```python
from build123d import *

# Parameters (mm, degrees)
SKETCH2_R           = 1.651
BOSS_EXTRUDE2_DEPTH = 6.35
FILLET2_R           = 20.32
FILLET3_R           = 2.54


with BuildPart() as part:
    # Sketch2 → Boss-Extrude2 (new body)
    with BuildSketch(Plane(origin=(0, 0, 0), x_dir=(0, 0, -1), z_dir=(1, 0, 0))):
        with BuildLine():
            Line((-22.16, -6.6675), (-22.16, -44.45))
            ThreePointArc((-22.16, -44.45), (0, -66.61), (22.16, -44.45))
            Line((22.16, -44.45), (22.16, 44.45))
            ThreePointArc((22.16, 44.45), (0, 66.61), (-22.16, 44.45))
            Line((-22.16, 44.45), (-22.16, 6.6675))
            Line((-22.16, 6.6675), (-126.3, 6.6675))
            Line((-126.3, 6.6675), (-126.3, -6.6675))
            Line((-126.3, -6.6675), (-22.16, -6.6675))
        make_face()
        with BuildLine():
            ThreePointArc((12, -44.45), (0, -56.45), (-12, -44.45))
            Line((-12, -44.45), (-12, 44.45))
            ThreePointArc((-12, 44.45), (0, 56.45), (12, 44.45))
            Line((12, 44.45), (12, -44.45))
        make_face(mode=Mode.SUBTRACT)
        with Locations((-111.06, 0)):
            Circle(SKETCH2_R, mode=Mode.SUBTRACT)
        with Locations((-103.44, 0)):
            Circle(SKETCH2_R, mode=Mode.SUBTRACT)
        with Locations((-118.68, 0)):
            Circle(SKETCH2_R, mode=Mode.SUBTRACT)
    extrude(amount=BOSS_EXTRUDE2_DEPTH)

    # Fillet2
    fillet2_edges = [part.edges().sort_by_distance(p)[0] for p in [
        (3.175, 6.6675, 22.16),
        (3.175, -6.6675, 22.16),
    ]]
    fillet(fillet2_edges, radius=FILLET2_R)

    # Fillet3
    fillet3_edges = [part.edges().sort_by_distance(p)[0] for p in [
        (3.175, 6.6675, 126.3),
        (3.175, -6.6675, 126.3),
    ]]
    fillet(fillet3_edges, radius=FILLET3_R)


solid = part.part
```
Check sheet for the modelled part. Datum: model origin and axes. Units: mm. A direction names the side the tool comes from. Give positions to 0.01 mm unless a question says otherwise; leave off trailing zeros. Order: outer loops, then holes, each group sorted by start corner. A loop starts at its lowest first (then second) coordinate and runs counter-clockwise, first axis right, second up. Notation, with made-up numbers: (73, 61) -> (114, 61) arc R18 cw to (114, 72) -> close; hole circle Ø2 at (-37, 37.25). An arc over 180 degrees is marked (long way). Use CSV: the item, a comma, the result in double quotes. Start each with the question number.
1) Sectioned sample at A-A, the plane z = 111.06. Record the boundary of the cut face in (x, y).
2) Set-up check for faces 1 (the face through (3, 0, 126.3)), 2 (the face through (0, 0, 25)), 3 (the face through (3, -36, 22.16)), 4 (the face through (3.131, -56.447, -0.264)), 5 (the face through (3, 36, 22.16)): record each of +Z, -Z, +X, -X, +Y, -Y from which the full face is reachable in a straight line by a thin tool's end or side.
3) Sectioned sample at D-D, the plane y = 0. Record the boundary of the cut face in (x, z), plus the area to 3 significant figures.
4) Sectioned sample at B-B, the plane y = -34.5. Record the boundary of the cut face in (x, z), plus the area to 3 significant figures.
5) Mould release check, pull along Z, two halves, no side actions. Record for faces 6 (the face through (3, 1, -12)), 7 (the face through (3, 6.668, 83)), 8 (the face through (3.22, -12.78, 27.95)): released by +Z, released by -Z, zero draft, split by the parting line, or undercut.
6) Material ranges on line 1 (Z direction, x = 4.5, y = -40.5); line 2 (Y direction, x = 3, z = 51); line 3 (Y direction, x = 4.5, z = 111.06), recorded low to high. Write a range as from..to.
7) Sectioned sample at C-C, the plane x = 3.75. Record the boundary of the cut face in (y, z).
8) Go/stop test with flat-tipped pins: P1, Ø2, axis at y = 0, z = 111.06, coming from the +X side; P2, Ø1.9, axis at x = 2, z = 80, coming from the -Y side; P3, Ø3, axis at x = 2.5, y = 33.5, coming from the +Z side; P4, Ø1.9, axis at x = 2, y = 18, coming from the +Z side. Record where each tip stops, or that it passes through.
Recorded:
1,outline,"(0, -6.67) -> (6.35, -6.67) -> (6.35, -1.65) -> (0, -1.65) -> close; (0, 1.65) -> (6.35, 1.65) -> (6.35, 6.67) -> (0, 6.67) -> close"
2,face 1,"+Z, +X, -X, +Y, -Y"
2,face 2,"+Z, -Z, -X, +Y, -Y"
2,face 3,"+Z, +X, -X, -Y"
2,face 4,"+X, -X"
2,face 5,"+Z, +X, -X, +Y"
3,outline,"(0, -22.16) -> (6.35, -22.16) -> (6.35, -12) -> (0, -12) -> close; (0, 12) -> (6.35, 12) -> (6.35, 101.79) -> (0, 101.79) -> close; (0, 105.09) -> (6.35, 105.09) -> (6.35, 109.41) -> (0, 109.41) -> close; (0, 112.71) -> (6.35, 112.71) -> (6.35, 117.03) -> (0, 117.03) -> close; (0, 120.33) -> (6.35, 120.33) -> (6.35, 126.3) -> (0, 126.3) -> close"
3,area,"727 mm2"
4,outline,"(0, -22.16) -> (6.35, -22.16) -> (6.35, -12) -> (0, -12) -> close; (0, 12) -> (6.35, 12) -> (6.35, 22.16) -> (0, 22.16) -> close"
4,area,"129 mm2"
5,face 6,"undercut"
5,face 7,"zero draft"
5,face 8,"released by +Z"
6,line 1,"-22.16..-12, 12..22.16"
6,line 2,"-6.67..6.67"
6,line 3,"-6.67..-1.65, 1.65..6.67"
7,outline,"(-44.45, -22.16) -> (44.45, -22.16) arc R22.16 ccw to (44.45, 22.16) -> (26.99, 22.16) arc R20.32 cw to (6.67, 42.48) -> (6.67, 123.76) arc R2.54 ccw to (4.13, 126.3) -> (-4.13, 126.3) arc R2.54 ccw to (-6.67, 123.76) -> (-6.67, 42.48) arc R20.32 cw to (-26.99, 22.16) -> (-44.45, 22.16) arc R22.16 ccw to start; hole (-44.45, -12) -> (44.45, -12) arc R12 ccw to (44.45, 12) -> (-44.45, 12) arc R12 ccw to start; hole circle Ø3.3 at (0, 103.44); hole circle Ø3.3 at (0, 111.06); hole circle Ø3.3 at (0, 118.68)"
8,P1,"through"
8,P2,"y = -6.67"
8,P3,"z = 22.16"
8,P4,"z = 24.76"
